from build123d import *

# Parameters (mm, degrees)
F0_R      = 27.5
F1_DEPTH  = 10
F2_DEPTH  = 20
F4_DEPTH  = 25
F5_W      = 40
F5_H      = 12
F6_DEPTH  = 7
F8_W      = 44.069208
F8_H      = 19.358708
F9_DEPTH  = 3
F7_W      = 24
F7_H      = 12
F10_DEPTH = 25
F11_R     = 1.5
F12_DEPTH = 25
F13_R     = 1.5
F14_DEPTH = 25


with BuildPart() as f1:
    # F0 (on Top) → F1 (new body)
    with BuildSketch(Plane.XY):
        with BuildLine():
            ThreePointArc((-12.5, 50.037254), (-27.025356, 26.362934), (-31.482419, -1.052282))
            ThreePointArc((-31.482419, -1.052282), (-24.455823, -19.853532), (-7.5, -30.594117))
            Line((-7.5, -30.594117), (-2.5, -30.712094))
            Line((-2.5, -30.712094), (2.5, -30.712094))
            Line((2.5, -30.712094), (7.5, -30.594117))
            ThreePointArc((7.5, -30.594117), (24.784067, -19.442222), (31.5, 0))
            Line((31.5, 0), (31.5, 50.037254))
            Line((31.5, 50.037254), (-12.5, 50.037254))
        make_face()
        Circle(F0_R, mode=Mode.SUBTRACT)
    extrude(amount=F1_DEPTH)

    # F0 (on Top) → F2 (join)
    with BuildSketch(Plane.XY):
        Polygon((7.5, -30.594117), (2.5, -30.712094), (2.5, -40.594117), (7.5, -40.594117), align=None)
        Polygon((-2.5, -30.712094), (-7.5, -30.594117), (-7.5, -40.594117), (-2.5, -40.594117), align=None)
    extrude(amount=F2_DEPTH)

    # F3 (on face) → F4 (cut)
    with BuildSketch(Plane(origin=(-7.5, 0, 0), x_dir=(0, -1, 0), z_dir=(-1, 0, 0))):
        Polygon((40.594117, 10), (30.594117, 0), (40.594117, 0), align=None)
    extrude(amount=-F4_DEPTH, mode=Mode.SUBTRACT)

    # F5 (on face) → F6 (cut)
    with BuildSketch(Plane.XY.offset(10)):
        with Locations((12.876151, 44.037254)):
            Rectangle(F5_W, F5_H)
    extrude(amount=-F6_DEPTH, mode=Mode.SUBTRACT)

    # F8 (on face) → F9 (join)
    with BuildSketch(Plane.XY):
        with Locations((9.436336, 40.292357)):
            Rectangle(F8_W, F8_H)
    extrude(amount=-F9_DEPTH)

    # F7 (on face) → F10 (cut)
    with BuildSketch(Plane.XY.offset(3)):
        with Locations((12.176151, 44.037254)):
            Rectangle(F7_W, F7_H)
    extrude(amount=-F10_DEPTH, mode=Mode.SUBTRACT)

    # F11 (on face) → F12 (cut)
    with BuildSketch(Plane.XY.offset(10)):
        with Locations((-15.985942, 34.45212)):
            Circle(F11_R)
    extrude(amount=-F12_DEPTH, mode=Mode.SUBTRACT)

    # F13 (on face) → F14 (cut)
    with BuildSketch(Plane(origin=(-7.5, 0, 0), x_dir=(0, -1, 0), z_dir=(-1, 0, 0))):
        with Locations((35.594117, 15)):
            Circle(F13_R)
    extrude(amount=-F14_DEPTH, mode=Mode.SUBTRACT)


solid = f1.part
CAD build for the part. Positions are in the model's coordinates, mm. A direction names the side the tool comes from. Round coordinates to 2 decimals unless told otherwise and drop trailing zeros. Loops run counter-clockwise (first coordinate to the right, second up) from the corner with the lowest first, then second, coordinate; pieces in that order, holes last. Notation, with made-up numbers: (70, 7) - (120, 7) arc R35 ccw to (120, 43) - close; hole circle Ø5 at (54, 67). An arc over 180 degrees is marked (long way). Put each result on its own line as item: value.
1. Slice it at A-A on z = 11.5. List the corners of the cut face in (x, y).
Geometry check:
outline: (-7.5, -40.59) - (-2.5, -40.59) - (-2.5, -30.71) - (-7.5, -30.59) - close; (2.5, -40.59) - (7.5, -40.59) - (7.5, -30.59) - (2.5, -30.71) - close
2. Wall check: line 1 (Y direction, x = -16, z = 9.25); line 2 (Y direction, x = 0, z = 5.5); line 3 (X direction, y = -31.5, z = 3.25). Give the ranges that are in metal, low to high.
Geometry check:
line 1: -27.13 to -22.37, 22.37 to 32.95, 35.95 to 45.94
line 2: -30.71 to -27.5, 27.5 to 38.04
line 3: -7.5 to -2.5, 2.5 to 7.5
3. Slice it at B-B on x = 11. List the corners of the cut face in (y, z).
Geometry check:
outline: (-29.52, 0) - (-25.2, 0) - (-25.2, 10) - (-29.52, 10) - close; (25.2, 0) - (30.61, 0) - (30.61, -3) - (38.04, -3) - (38.04, 10) - (25.2, 10) - close
4. Two-plate mould, pull along Z, no slides. Class faces 1 (the flat face through (4, 36, -3)), 2 (the cylindrical face through (4.965, -37.025, 15.451)), 3 (the flat face through (28, 50.037, 1)): released by +Z, released by -Z, zero draft, split by the parting line, or undercut.
Geometry check:
face 1: released by -Z
face 2: undercut
face 3: zero draft
5. Slice it at D-D on z = 1.75. List the corners of the cut face in (x, y), and give its area (3 significant figures).
Geometry check:
outline: (-31.48, -1.05) arc R31.5 ccw to (-7.5, -30.59) - (-7.5, -32.34) - (-2.5, -32.34) - (-2.5, -30.71) - (2.5, -30.71) - (2.5, -32.34) - (7.5, -32.34) - (7.5, -30.59) arc R31.5 ccw to (31.5, 0) - (31.5, 50.04) - (24.18, 50.04) - (24.18, 38.04) - (0.18, 38.04) - (0.18, 50.04) - (-12.5, 50.04) arc R71.83 ccw to start; hole circle Ø55 at (0, 0); hole circle Ø3 at (-15.99, 34.45)
area: 1,760 mm²
6. Pin check, flat tips, straight feed: P1, Ø5, axis at y = 43.5, z = -1, coming from the -X side; P2, Ø3, axis at y = -36, z = 12, coming from the +X side; P3, Ø12, axis at x = -17, z = 4, coming from the -Y side; P4, Ø12, axis at x = 2, y = 28, coming from the -Z side. Stop position of each tip, or through.
Geometry check:
P1: x = -19.45
P2: x = 7.5
P3: y = -29.52
P4: z = -3
7. Slice it at C-C on y = 6. List the corners of the cut face in (x, z), and give its area (3 significant figures).
Geometry check:
outline: (-31.37, 0) - (-26.84, 0) - (-26.84, 10) - (-31.37, 10) - close; (26.84, 0) - (31.5, 0) - (31.5, 10) - (26.84, 10) - close
area: 92.0 mm²
8. 3-axis set-ups, long thin cutter, end or side, ignore diameter. For faces 4 (the flat face through (9, 30.613, -1)), 5 (the flat face through (-5, -40.594, 15)), 6 (the flat face through (-2.5, -35, 12)): which of +Z, -Z, +X, -X, +Y, -Y reach the whole face in a straight line?
Geometry check:
face 4: -Z, +X, -X, -Y
face 5: +Z, -Z, +X, -X, -Y
face 6: +Z, -Z, -Y
